Autodesk Inventor part; units mm, degrees
ref_plane "YZ Plane" through (0, 0, 0) normal (1, 0, 0) x (0, 1, 0)
ref_plane "XZ Plane" through (0, 0, 0) normal (0, 1, 0) x (-1, 0, 0)
ref_plane "XY Plane" through (0, 0, 0) normal (0, 0, 1) x (1, 0, 0)
sketch "Sketch9" plane through (0, 0, 0) normal (0, 1, 0) x (-1, 0, 0)
  line L0 (15, 15) -> (-15, 15)
  line L1 (-15, 15) -> (-15, -15)
  line L2 (-15, -15) -> (15, -15)
  line L3 (15, -15) -> (15, 15)
  line L4 (15, 15) -> (-15, -15) construction
  line L5 (-15, 15) -> (15, -15) construction
  line L6 (-13, 13) -> (13, 13)
  line L7 (13, 13) -> (13, -13)
  line L8 (13, -13) -> (-13, -13)
  line L9 (-13, -13) -> (-13, 13)
  point P0 (0, 0)
  dimension "d172" = 30
  dimension "d173" = 30
  dimension "d174" = 2
extrude "Extrusion3" add sketch "Sketch9" against normal blind 500
sketch "Sketch10" plane through (0, 0, 0) normal (1, 0, 0) x (0, 1, 0)
  line L0 (0, 15) -> (0, -15) construction
  line L1 (0, 15) -> (-500, 15) construction
  line L2 (-500, -15) -> (-500, 15) construction
  line L3 (0, -15) -> (-500, -15) construction
  line L4 (-68.5, 8.5) -> (-51.5, 8.5)
  line L5 (-51.5, 8.5) -> (-51.5, -8.5)
  line L6 (-51.5, -8.5) -> (-68.5, -8.5)
  line L7 (-68.5, -8.5) -> (-68.5, 8.5)
  line L8 (-68.5, 8.5) -> (-51.5, -8.5) construction
  line L9 (-51.5, 8.5) -> (-68.5, -8.5) construction
  line L10 (-218.5, 8.5) -> (-201.5, 8.5)
  line L11 (-201.5, 8.5) -> (-201.5, -8.5)
  line L12 (-201.5, -8.5) -> (-218.5, -8.5)
  line L13 (-218.5, -8.5) -> (-218.5, 8.5)
  line L14 (-218.5, 8.5) -> (-201.5, -8.5) construction
  line L15 (-201.5, 8.5) -> (-218.5, -8.5) construction
  line L16 (-368.5, 8.5) -> (-351.5, 8.5)
  line L17 (-351.5, 8.5) -> (-351.5, -8.5)
  line L18 (-351.5, -8.5) -> (-368.5, -8.5)
  line L19 (-368.5, -8.5) -> (-368.5, 8.5)
  line L20 (-368.5, 8.5) -> (-351.5, -8.5) construction
  line L21 (-351.5, 8.5) -> (-368.5, -8.5) construction
  circle A0 centre (-470, 0) radius 8.5
  line L22 (0, 0) -> (30, 0)
  circle A1 centre (-60, 0) radius 8.5
  circle A2 centre (-210, 0) radius 8.5
  circle A3 centre (-360, 0) radius 8.5
  dimension "d177" = 17
  dimension "d178" = 17
  dimension "d181" = 30
  dimension "d182" = 90
  dimension "d183" = 240
  dimension "d184" = 390
  dimension "d185" = 500
  dimension "d186" = 17
extrude "Extrusion4" cut sketch "Sketch10" along normal through all contours A1 | A2 | A3 | A0
properties part number "PNS 754 FDS 1200 way tube 1" material "Stainless Steel"
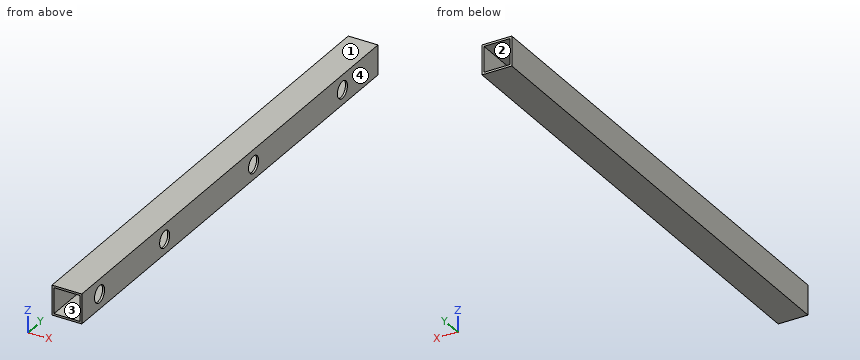
Here's how the part is built. I have some questions about the finished solid (model axes, mm). Face numbers are marked on the shaded views. Coordinates: 2 decimals unless noted, no trailing zeros. Write each loop counter-clockwise with the first axis right and the second up, starting at its lowest first coordinate (ties: lowest second). Pieces come first, ordered by that corner, then holes.
Item 1: I want a section at B-B on z = 0. Write out the boundary of the cut face in (x, y).
Item 2: If we mould it in two halves opening along X, with no side actions, what happens to the marked faces 1, 2, 3 and 4? For each: +X half, -X half, draft (parallel to the pull), parting line (faces both ways), or undercut.
Item 3: If I drill on line 1 (Y direction, x = 13.45, z = 0); line 2 (Z direction, x = 14.5, y = -210); line 3 (Z direction, x = 4.5, y = -445.5), over which ranges is the centre line in solid material (lowest first)?
Item 4: Will this pin go through, and if not, where does the flat tip stop? pin 1 (10 mm diameter, centred on y = -470, z = 0, fed in from +X).
Item 5: I want a section at C-C on y = -360. Write out the boundary of the cut face in (x, z).
Item 6: I want a section at A-A on y = -292. Write out the boundary of the cut face in (x, z).
Findings below:
1. outline: (-15, -500) - (-13, -500) - (-13, 0) - (-15, 0) - close; (13, -500) - (15, -500) - (15, -478.5) - (13, -478.5) - close; (13, -461.5) - (15, -461.5) - (15, -368.5) - (13, -368.5) - close; (13, -351.5) - (15, -351.5) - (15, -218.5) - (13, -218.5) - close; (13, -201.5) - (15, -201.5) - (15, -68.5) - (13, -68.5) - close; (13, -51.5) - (15, -51.5) - (15, 0) - (13, 0) - close
2. face 1: draft
2. face 2: undercut
2. face 3: undercut
2. face 4: +X half
3. line 1: y = -500 to -478.5, -461.5 to -368.5, -351.5 to -218.5, -201.5 to -68.5, -51.5 to 0
3. line 2: z = -15 to -8.5, 8.5 to 15
3. line 3: z = -15 to -13, 13 to 15
4. pin 1: stops at x = -13
5. outline: (-15, -15) - (15, -15) - (15, -8.5) - (13, -8.5) - (13, -13) - (-13, -13) - (-13, 13) - (13, 13) - (13, 8.5) - (15, 8.5) - (15, 15) - (-15, 15) - close
6. outline: (-15, -15) - (15, -15) - (15, 15) - (-15, 15) - close; hole (-13, -13) - (13, -13) - (13, 13) - (-13, 13) - close
